```python
from build123d import *

# Parameters (mm, degrees)
SKETCH1_W                = 35
SKETCH1_H                = 60
BOSS_EXTRUDE1_DEPTH      = 20
FILLET1_R                = 2
BOSS_EXTRUDE2_DEPTH      = 3
BOSS_EXTRUDE2_DEPTH_BACK = 3
SKETCH2_R                = 10
SKETCH3_R                = 6
CUT_EXTRUDE1_DEPTH       = 1


with BuildPart() as part:
    # Sketch1 → Boss-Extrude1 (new body)
    with BuildSketch(Plane(origin=(0, 0, 0), x_dir=(1, 0, 0), z_dir=(0, 1, 0))):
        Rectangle(SKETCH1_W, SKETCH1_H)
    extrude(amount=BOSS_EXTRUDE1_DEPTH)

    # Fillet1
    fillet1_edges = [part.edges().sort_by_distance(p)[0] for p in [
        (-17.5, 20, 0),
        (0, 20, 30),
        (17.5, 20, 0),
        (0, 0, 30),
        (-17.5, 0, 0),
        (0, 0, -30),
        (17.5, 0, 0),
        (0, 20, -30),
        (17.5, 10, 30),
        (-17.5, 10, 30),
        (-17.5, 10, -30),
        (17.5, 10, -30),
    ]]
    fillet(fillet1_edges, radius=FILLET1_R)

    # Sketch2 → Boss-Extrude2 (add, two sides: drawn at the far end of the back side and taken through both)
    with BuildSketch(Plane(origin=(0, 0, -30), x_dir=(-1, 0, 0), z_dir=(0, 0, -1)).offset(-BOSS_EXTRUDE2_DEPTH_BACK)):
        with Locations((5, 10)):
            Circle(SKETCH2_R)
    extrude(amount=BOSS_EXTRUDE2_DEPTH + BOSS_EXTRUDE2_DEPTH_BACK)

    # Sketch3 → Cut-Extrude1 (cut)
    with BuildSketch(Plane(origin=(0, 0, -33), x_dir=(-1, 0, 0), z_dir=(0, 0, -1))):
        with Locations((5, 10)):
            Circle(SKETCH3_R)
    extrude(amount=-CUT_EXTRUDE1_DEPTH, mode=Mode.SUBTRACT)


solid = part.part
```
Geometry check sheet. Reference: the model listing, model coordinates, mm. A direction names the side the tool comes from. Give positions to 0.01 mm unless a question says otherwise; leave off trailing zeros. Order: outer loops, then holes, each group sorted by start corner. A loop starts at its lowest first (then second) coordinate and runs counter-clockwise, first axis right, second up.
1. Release check for a two-part mould opening along X. For faces 5 (the face through (-5, 3, -33)), 6 (the face through (-5, 10, -32)), 7 (the face through (16.93, 0.6, -0.39)), 8 (the face through (-3.699, 4.143, -32.507)) record: pulls with the +X half, pulls with the -X half, needs draft (parallel to the pull), parting line crosses it, or undercut.
2. Section check A-A, the plane x = 6. Enter the section's corners in (y, z), and give its area (3 significant figures).
3. Thickness scan on L1, parallel to Y at x = -5, z = -32.2; L2, parallel to Z at x = 15, y = 11.25; L3, parallel to Z at x = -2, y = 11.5. Record the ranges inside material, lowest first.
4. Section check C-C, the plane y = 5. Enter the section's corners in (x, z), and give its area (3 significant figures).
5. Access from +Z, -Z, +X, -X, +Y, -Y to the whole of each face (thin tool, end or side, straight path). Record for faces 1 (the face through (7.67, 19.4, -29.43)), 2 (the face through (-15.3, 10, -30)), 3 (the face through (-11.3, 0.4, -29.2)), 4 (the face through (7.67, 0.6, -29.43)).
6. Section check B-B, the plane y = 10. Enter the section's corners in (x, z).
7. Gauge pin test, flat end, axial feed: pin 1 Ø8 at (x, y) = (8, 16) entering from -Z. Record the tip position at first contact, or that the pin passes through.
8. Section check D-D, the plane y = 19.25. Enter the section's corners in (x, z).
Values follow:
1. face 5: needs draft
1. face 6: undercut
1. face 7: pulls with the +X half
1. face 8: undercut
2. outline: (0, -28) arc R2 ccw to (2, -30) - (18, -30) arc R2 ccw to (20, -28) - (20, 28) arc R2 ccw to (18, 30) - (2, 30) arc R2 ccw to (0, 28) - close
2. area: 1,200 mm2
3. L1: y = 0 to 4, 16 to 20
3. L2: z = -30 to 30
3. L3: z = -32 to 30
4. outline: (-17.5, -28) arc R2 ccw to (-15.5, -30) - (-13.66, -30) - (-13.66, -33) - (-8.32, -33) - (-8.32, -32) - (-1.68, -32) - (-1.68, -33) - (3.66, -33) - (3.66, -30) - (15.5, -30) arc R2 ccw to (17.5, -28) - (17.5, 28) arc R2 ccw to (15.5, 30) - (-15.5, 30) arc R2 ccw to (-17.5, 28) - close
4. area: 2,140 mm2
5. face 1: -Z, +X, +Y
5. face 2: -Z, -X
5. face 3: -Z, -X, -Y
5. face 4: -Z, +X, -Y
6. outline: (-17.5, -28) arc R2 ccw to (-15.5, -30) - (-15, -30) - (-15, -33) - (-11, -33) - (-11, -32) - (1, -32) - (1, -33) - (5, -33) - (5, -30) - (15.5, -30) arc R2 ccw to (17.5, -28) - (17.5, 28) arc R2 ccw to (15.5, 30) - (-15.5, 30) arc R2 ccw to (-17.5, 28) - close
7. pin 1: stops at z = -30
8. outline: (-17.06, -28) arc R1.56 ccw to (-15.5, -29.56) - (-8.8, -29.56) - (-8.8, -33) - (-1.2, -33) - (-1.2, -29.56) - (15.5, -29.56) arc R1.56 ccw to (17.06, -28) - (17.06, 28) arc R1.56 ccw to (15.5, 29.56) - (-15.5, 29.56) arc R1.56 ccw to (-17.06, 28) - close
